Could you check a few things on this model? Use its own coordinates, in mm. Face numbers are marked on the shaded views. A direction names the side the tool comes from. Coordinates: 2 decimals unless noted, no trailing zeros. Write each loop counter-clockwise with the first axis right and the second up, starting at its lowest first coordinate (ties: lowest second). Pieces come first, ordered by that corner, then holes.
```python
from build123d import *

# Parameters (mm, degrees)
F0_R           = 8
F1_DEPTH       = 10
F1_TAPER       = 10
F3_DEPTH       = 25
F5_D           = 4.4
F5_CBORE_D     = 8.25
F5_CBORE_DEPTH = 4
F7_D           = 5
F9_DEPTH       = 12.5
F10_R          = 1


with BuildPart() as f1:
    # F0 (on Top) → F1 (new body)
    with BuildSketch(Plane.XY):
        Circle(F0_R)
    extrude(amount=F1_DEPTH, taper=F1_TAPER)

    # F2 (on face) → F3 (cut)
    with BuildSketch(Plane(origin=(0, 0, 0), x_dir=(1, 0, 0), z_dir=(0, 0, -1))):
        with BuildLine():
            ThreePointArc((8, 0), (7.3484692283, 3.1622776602), (5.5, 5.8094750193))
            Line((5.5, 5.8094750193), (5.5, -5.8094750193))
            ThreePointArc((5.5, -5.8094750193), (7.3484692283, -3.1622776602), (8, 0))
        make_face()
    extrude(amount=-F3_DEPTH, mode=Mode.SUBTRACT)

    # F5 (through all)
    with Locations(Plane.XY.offset(10)):
        with Locations((-1.5, 0)):
            CounterBoreHole(F5_D / 2, F5_CBORE_D / 2, F5_CBORE_DEPTH)

    # F7 (through all)
    with Locations(Plane.XY.offset(10)):
        with Locations((7, 0)):
            Hole(F7_D / 2)

    # F8 (on Front) → F9 (cut, symmetric)
    with BuildSketch(Plane.XZ):
        with BuildLine():
            Line((10.4339603065, 10), (3.5, 10))
            Line((3.5, 10), (5.4315959713, 9.2969565618))
            ThreePointArc((5.4315959713, 9.2969565618), (5.5563771079, 9.1607818467), (5.5164008313, 8.9804605157))
            Line((5.5164008313, 8.9804605157), (2.6557981563, 5.5713270008))
            Line((2.6557981563, 5.5713270008), (5.4315959713, 4.5610192198))
            ThreePointArc((5.4315959713, 4.5610192198), (5.5563771079, 4.4248445046), (5.5164008313, 4.2445231737))
            Line((5.5164008313, 4.2445231737), (0.7803240521, -1.3997133427))
            Line((0.7803240521, -1.3997133427), (10.4339603065, -1.3997133427))
            Line((10.4339603065, -1.3997133427), (10.4339603065, 10))
        make_face()
    extrude(amount=F9_DEPTH, both=True, mode=Mode.SUBTRACT)

    # F10
    f10_edges = [f1.edges().sort_by_distance(p)[0] for p in [
        (2.655798, 0, 5.571327),
    ]]
    fillet(f10_edges, radius=F10_R)


solid = f1.part
```
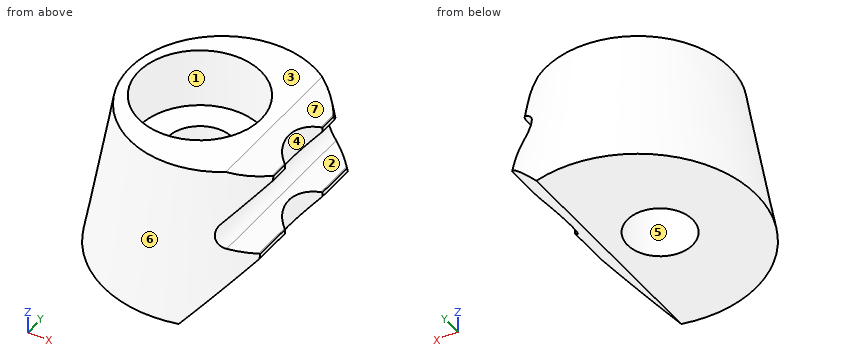
1. I want a section at A-A on y = 0. Please give me the cut outline in (x, z) (3 decimals).
Verdict:
outline: (-8, 0) - (-3.7, 0) - (-3.7, 6) - (-5.625, 6) - (-5.625, 10) - (-6.237, 10) - close; (0.7, 0) - (1.955, 0) - (4.5, 3.033) - (4.5, 4.9) - (3.998, 5.083) arc R1 cw to (3.574, 6.665) - (4.5, 7.769) - (4.5, 9.636) - (3.5, 10) - (2.625, 10) - (2.625, 6) - (0.7, 6) - close
2. I want a section at C-C on z = 4. Please give me the cut outline in (x, y), plus the area to 3 significant figures.
Verdict:
outline: (5.31, -5) - (5.31, -1.84) arc R2.5 cw to (5.31, 1.84) - (5.31, 5) arc R7.29 ccw (long way) to start; hole circle Ø4.4 at (-1.5, 0)
area: 136 mm2
3. I want a section at D-D on z = 5.5. Please give me the cut outline in (x, y), plus the area to 3 significant figures.
Verdict:
outline: (3.49, -6.1) - (3.49, 6.1) arc R7.03 ccw (long way) to start; hole circle Ø4.4 at (-1.5, 0)
area: 109 mm2
4. I want a section at B-B on x = 0. Please give me the cut outline in (y, z), plus the area to 3 significant figures.
Verdict:
outline: (-8, 0) - (-1.61, 0) - (-1.61, 6) - (-3.84, 6) - (-3.84, 10) - (-6.24, 10) - close; (1.61, 0) - (8, 0) - (6.24, 10) - (3.84, 10) - (3.84, 6) - (1.61, 6) - close
area: 92.3 mm2
5. For pin 1 (1.5 mm diameter, centred on y = -0.5, z = 4, fed in from -X); pin 2 (5 mm diameter, centred on x = -1.5, y = 0, fed in from +Z); pin 3 (2 mm diameter, centred on y = 4.5, z = 3.5, fed in from -X); pin 4 (3.5 mm diameter, centred on x = -1.5, y = 0, fed in from +Z), each with a flat end and sliding along its axis, tell me the tip position at first contact or that it passes through.
Verdict:
pin 1: stops at x = -7.42
pin 2: stops at z = 6
pin 3: stops at x = -6.54
pin 4: passes through
6. On a 3-axis mill with a long thin cutter (end or side, diameter ignored), from which of +Z, -Z, +X, -X, +Y, -Y can I reach the whole of each face in a straight line? I mean the marked faces 1, 2 and 3. Say none if no direction works.
Verdict:
face 1: +Z
face 2: +X, +Y, -Y
face 3: +Z, +X, -X, +Y, -Y
7. Please list where these lines run through material, in increasing order: line 1 along Z through (x, y) = (-3.75, 3); line 2 along Y through (x, z) = (-0.25, 8.5); line 3 along Y through (x, z) = (-1.5, 8.55) (3 decimals).
Verdict:
line 1: z = 0 to 6
line 2: y = -6.5 to -3.93, 3.93 to 6.5
line 3: y = -6.317 to -4.125, 4.125 to 6.317
8. If we mould it in two halves opening along Y, with no side actions, what happens to the marked faces 4, 5, 6 and 7? For each: pulls with the +Y half, pulls with the -Y half, needs draft (parallel to the pull), parting line crosses it, or undercut.
Verdict:
face 4: undercut
face 5: undercut
face 6: parting line crosses it
face 7: needs draft
